from build123d import *

# Parameters (mm, degrees)
SKETCH2_R           = 2
BOSS_EXTRUDE1_DEPTH = 11.6
SKETCH3_R           = 4
BOSS_EXTRUDE2_DEPTH = 0.3
SKETCH4_R           = 8
BOSS_EXTRUDE3_DEPTH = 0.7
SKETCH5_R           = 1.5
CUT_EXTRUDE1_DEPTH  = 8.5
SKETCH7_R           = 1.5
CUT_EXTRUDE2_DEPTH  = 17.419805115
CHAMFER1_SIZE       = 0.1


with BuildPart() as part:
    # Sketch2 → Boss-Extrude1 (new body)
    with BuildSketch(Plane.XY):
        Circle(SKETCH2_R)
    extrude(amount=BOSS_EXTRUDE1_DEPTH)

    # Sketch3 → Boss-Extrude2 (add)
    with BuildSketch(Plane.XY.offset(11.6)):
        Circle(SKETCH3_R)
    extrude(amount=BOSS_EXTRUDE2_DEPTH)

    # Sketch4 → Boss-Extrude3 (add)
    with BuildSketch(Plane.XY.offset(11.9)):
        Circle(SKETCH4_R)
    extrude(amount=BOSS_EXTRUDE3_DEPTH)

    # Sketch5 → Cut-Extrude1 (cut)
    with BuildSketch(Plane(origin=(0, 0, 0), x_dir=(-1, 0, 0), z_dir=(0, 0, -1))):
        Circle(SKETCH5_R)
    extrude(amount=-CUT_EXTRUDE1_DEPTH, mode=Mode.SUBTRACT)

    # Sketch7 → Cut-Extrude2 (cut, through all)
    with BuildSketch(Plane(origin=(0, 0, 11.9), x_dir=(-1, 0, 0), z_dir=(0, 0, -1))):
        with Locations((0, -6)):
            Circle(SKETCH7_R)
    extrude(amount=-CUT_EXTRUDE2_DEPTH, mode=Mode.SUBTRACT)

    # Chamfer1
    chamfer1_edges = [part.edges().sort_by_distance(p)[0] for p in [
        (-8, 0, 12.6),
        (-2, 0, 0),
        (-8, 0, 11.9),
    ]]
    chamfer(chamfer1_edges, length=CHAMFER1_SIZE)


solid = part.part
Can you work these out from the model? Positions are in its coordinate system, mm. A direction names the side the tool comes from. Coordinates: 2 decimals unless noted, no trailing zeros. Write each loop counter-clockwise with the first axis right and the second up, starting at its lowest first coordinate (ties: lowest second). Pieces come first, ordered by that corner, then holes. Notation, with made-up numbers: (26.5, 62.25) -> (85.5, 62.25) arc R28 cw to (85.5, 101.25) -> close; hole circle Ø3 at (41, 2). An arc over 180 degrees is marked (long way). Write each question's results on one line, items separated by ' | '. Start each with the question number.
Q1. Imagine slicing it at B-B (z = 4.75). Write out the boundary of the cut face in (x, y), then the cut area to 3 significant figures.
Q2. I'm going to push flat-ended pins straight in: pin 1 (5 mm diameter, centred on y = -5, z = 3, fed in from +X); pin 2 (5 mm diameter, centred on y = -4, z = 11, fed in from -X); pin 3 (2 mm diameter, centred on y = 2, z = 1.5, fed in from +X); pin 4 (1.5 mm diameter, centred on x = 0.5, y = -0.5, fed in from -Z). Where does each tip first touch, or does it pass through?
Q3. Imagine slicing it at C-C (y = 0). Write out the boundary of the cut face in (x, z).
Q4. On a 3-axis mill with a long thin cutter (end or side, diameter ignored), from which of +Z, -Z, +X, -X, +Y, -Y can I reach the whole of each face in a straight line? I mean faces 1 (the face through (0.325, -7.464, 12.245)), 2 (the face through (0, 0, 8.5)). Say none if no direction works.
Q5. Imagine slicing it at A-A (x = 0). Write out the boundary of the cut face in (y, z).
Q6. Imagine slicing it at D-D (z = 9.5). Write out the boundary of the cut face in (x, y), then the cut area to 3 significant figures.
Q7. If I drill on probe 1 along Y at (x, z) = (0, 12.1); probe 2 along Z at (x, y) = (1.25, 7.5); probe 3 along Y at (x, z) = (0, 6), over which ranges is the centre line in solid material (lowest first)?
Q8. We'd pull the mould along X, two halves only. Please class faces 3 (the face through (-2, -1, 11.6)), 4 (the face through (0, -2, 6)), 5 (the face through (1.5, 0.07, 4.19)): +X half, -X half, draft (parallel to the pull), parting line (faces both ways), or undercut.
Taken from the geometry:
1) outline: circle Ø4 at (0, 0); hole circle Ø3 at (0, 0) | area: 5.50 mm^2
2) pin 1: passes through | pin 2: stops at x = -7.82 | pin 3: stops at x = 1.73 | pin 4: stops at z = 8.5
3) outline: (-8, 12) -> (-7.9, 11.9) -> (-4, 11.9) -> (-4, 11.6) -> (-2, 11.6) -> (-2, 0.1) -> (-1.9, 0) -> (-1.5, 0) -> (-1.5, 8.5) -> (1.5, 8.5) -> (1.5, 0) -> (1.9, 0) -> (2, 0.1) -> (2, 11.6) -> (4, 11.6) -> (4, 11.9) -> (7.9, 11.9) -> (8, 12) -> (8, 12.5) -> (7.9, 12.6) -> (-7.9, 12.6) -> (-8, 12.5) -> close
4) face 1: +Z, -Z | face 2: -Z
5) outline: (-8, 12) -> (-7.9, 11.9) -> (-7.5, 11.9) -> (-7.5, 12.6) -> (-7.9, 12.6) -> (-8, 12.5) -> close; (-4.5, 11.9) -> (-4, 11.9) -> (-4, 11.6) -> (-2, 11.6) -> (-2, 0.1) -> (-1.9, 0) -> (-1.5, 0) -> (-1.5, 8.5) -> (1.5, 8.5) -> (1.5, 0) -> (1.9, 0) -> (2, 0.1) -> (2, 11.6) -> (4, 11.6) -> (4, 11.9) -> (7.9, 11.9) -> (8, 12) -> (8, 12.5) -> (7.9, 12.6) -> (-4.5, 12.6) -> close
6) outline: circle Ø4 at (0, 0) | area: 12.6 mm^2
7) probe 1: y = -8 to -7.5, -4.5 to 8 | probe 2: z = 11.9 to 12.6 | probe 3: y = -2 to -1.5, 1.5 to 2
8) face 3: draft | face 4: parting line | face 5: undercut
